Source: three-view drawing plus pictorial views. Frame: mm from the lowest corner of the part. Coordinates: 2 decimals unless noted, no trailing zeros. Write each loop counter-clockwise with the first axis right and the second up, starting at its lowest first coordinate (ties: lowest second). Pieces come first, ordered by that corner, then holes. Notation, with made-up numbers: (-37, 86.5) - (-18, 86.5) arc R28 cw to (-18, 118.5) - close; hole circle Ø1 at (13, 76). An arc over 180 degrees is marked (long way). One line per item, written item: value.
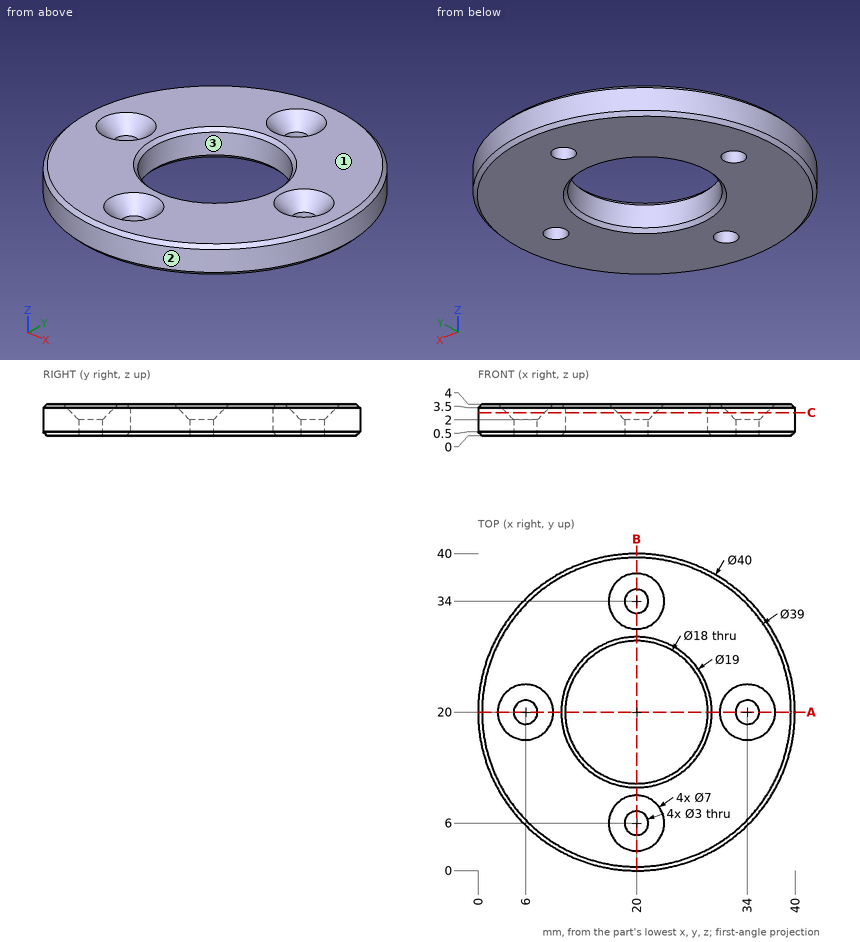
1) Section query C-C on z = 2.9. Output: boundary loops of the cut face in (x, y), then the cut area to 3 significant figures.
Values found:
outline: circle Ø40 at (20, 20); hole circle Ø4.8 at (6, 20); hole circle Ø18 at (20, 20); hole circle Ø4.8 at (20, 6); hole circle Ø4.8 at (20, 34); hole circle Ø4.8 at (34, 20)
area: 930 mm2
2) Draft query along X for the marked faces 1, 2 and 3. Return one class per face: released by +X, released by -X, zero draft, split by the parting line, or undercut.
Values found:
face 1: zero draft
face 2: split by the parting line
face 3: undercut
3) Section query A-A on y = 20. Output: boundary loops of the cut face in (x, z).
Values found:
outline: (0, 0.5) - (0.5, 0) - (4.5, 0) - (4.5, 2) - (2.5, 4) - (0.5, 4) - (0, 3.5) - close; (7.5, 0) - (10.5, 0) - (11, 0.5) - (11, 3.5) - (10.5, 4) - (9.5, 4) - (7.5, 2) - close; (29, 0.5) - (29.5, 0) - (32.5, 0) - (32.5, 2) - (30.5, 4) - (29.5, 4) - (29, 3.5) - close; (35.5, 0) - (39.5, 0) - (40, 0.5) - (40, 3.5) - (39.5, 4) - (37.5, 4) - (35.5, 2) - close
4) Contact query for flat-ended pins moving along their axis: P1, Ø3.5, axis at x = 34, y = 20, coming from the -Z side; P2, Ø11, axis at x = 20, y = 20, coming from the -Z side; P3, Ø1, axis at y = 31.5, z = 0.5, coming from the -X side; P4, Ø2, axis at x = 26.5, z = 3, coming from the -Y side. Output: stop coordinate, or through.
Values found:
P1: z = 0
P2: through
P3: x = 3.3
P4: y = 0.77
5) Material intervals for line 1 (Y direction, x = 20, z = 1.5); line 2 (Y direction, x = 21, z = 3.55); line 3 (X direction, y = 24, z = 0.4), sorted ascending.
Values found:
line 1: 0 to 4.5, 7.5 to 11, 29 to 32.5, 35.5 to 40
line 2: 0.08 to 3.12, 8.88 to 11.01, 28.99 to 31.12, 36.88 to 39.92
line 3: 0.51 to 11.83, 28.17 to 39.49
